```python
from build123d import *

# Parameters (mm, degrees)
F1_DEPTH = 2
F2_W     = 10
F2_H     = 3
F3_DEPTH = 10
F4_R     = 145
F5_DEPTH = 25
F6_R     = 2


with BuildPart() as f1:
    # F0 (on Top) → F1 (new body)
    with BuildSketch(Plane.XY):
        with BuildLine():
            Line((50, 15), (-50, 15))
            Line((-50, 15), (-50, -15))
            Line((-50, -15), (-40, -15))
            ThreePointArc((-40, -15), (-39.2634671, -7.3593095017), (-37.0809924355, 0))
            Line((-37.0809924355, 0), (37.0809924355, 0))
            ThreePointArc((37.0809924355, 0), (39.2634671, -7.3593095017), (40, -15))
            Line((40, -15), (50, -15))
            Line((50, -15), (50, 15))
        make_face()
    extrude(amount=F1_DEPTH)

    # F2 (on face) → F3 (join)
    with BuildSketch(Plane.XY.offset(2)):
        with Locations((-45, -13.5)):
            Rectangle(F2_W, F2_H)
        with Locations((45, -13.5)):
            Rectangle(F2_W, F2_H)
    extrude(amount=F3_DEPTH)

    # F4 (on Front) → F5 (cut)
    with BuildSketch(Plane.XZ):
        with Locations((0, 145)):
            Circle(F4_R)
    extrude(amount=F5_DEPTH, mode=Mode.SUBTRACT)

    # F6
    f6_edges = [f1.edges().sort_by_distance(p)[0] for p in [
        (-50, -13.5, 8.893424),
        (50, -13.5, 8.893424),
        (-40, -13.5, 5.626401),
        (40, -13.5, 5.626401),
        (37.080992, 0, 1),
        (-37.080992, 0, 1),
        (-50, 15, 1),
        (50, 15, 1),
    ]]
    fillet(f6_edges, radius=F6_R)


solid = f1.part
```
Design review of the part built by this model. Coordinates are the model's own, in mm. A direction names the side the tool comes from. Give positions to 0.01 mm unless a question says otherwise; leave off trailing zeros. Order: outer loops, then holes, each group sorted by start corner. A loop starts at its lowest first (then second) coordinate and runs counter-clockwise, first axis right, second up. Notation, with made-up numbers: M -38,79.5 L 10,79.5 A38 cw 10,118.5 Z; hole C 9,86.5 d3. An arc over 180 degrees is marked long. One line per question, with ' | ' between items. Start each with the question number.
Q1. We need section C-C (z = 5). Write out the cut boundary in (x, y), plus the area to 3 significant figures.
Q2. Machinability: for faces 4 (the face through (39.375, -7.956, 0.986)), 5 (the face through (45, -15, 3)), 6 (the face through (44.357, -13.479, 6.951)), which of the approach directions +Z, -Z, +X, -X, +Y, -Y give a long, thin tool a straight path to every point of the face, cutting with its end or side? Answer none if there is none.
Q3. We need section B-B (y = -6.25). Write out the cut boundary in (x, z).
Q4. We need section D-D (x = 14). Write out the cut boundary in (y, z).
Q5. The part is to be moulded in two halves that separate along X. For faces 1 (the face through (-44.44, -13.48, 6.98)), 2 (the face through (49.43, 14.4, 1.01)), 3 (the face through (-45, -12, 4)), say which applies: +X half, -X half, draft (parallel to the pull), parting line (faces both ways), or undercut.
Q6. For pin 1 Ø15 at (x, y) = (-10.5, 5) entering from +Z; pin 2 Ø3 at (x, z) = (-44, 6) entering from +Y; pin 3 Ø2 at (x, z) = (4.5, 1.5) entering from -Y, all flat-tipped, find the tip position at first contact; note any pin that passes through.
Q7. We need section A-A (z = 1). Write out the cut boundary in (x, y).
Q8. For L1, parallel to Z at x = 4, y = 3; L2, parallel to X at y = -2.5, z = 1; L3, parallel to X at y = -0.25, z = 1.75, list the stretches that pass through material, from the lowest coordinate up. Write a range as [from, to].
Returned:
1) outline: M -50,-15 L -40.2,-15 L -40.2,-12 L -50,-12 Z; M 40.2,-15 L 50,-15 L 50,-12 L 40.2,-12 Z | area: 58.8 mm2
2) face 4: +Z, -Z, -Y | face 5: +Z, -Z, +X, -X, -Y | face 6: +Z, +Y, -Y
3) outline: M -50,0 L -39.03,0 L -39.03,2 L -50,2 Z; M 39.03,0 L 50,0 L 50,2 L 39.03,2 Z
4) outline: M 0,0 L 15,0 L 15,2 L 0,2 Z
5) face 1: undercut | face 2: +X half | face 3: draft
6) pin 1: z = 2 | pin 2: y = -12 | pin 3: y = 0
7) outline: M -50,-15 L -40,-15 A40 cw -37.59,-1.32 A2 cw -35.71,0 L 35.71,0 A2 cw 37.59,-1.32 A40 cw 40,-15 L 50,-15 L 50,13 A2 ccw 48,15 L -48,15 A2 ccw -50,13 Z
8) L1: [0, 2] | L2: [-50, -38], [38, 50] | L3: [-50, -36.68], [36.68, 50]
